Source: CAD feature listing. Evaluate the final solid. Frame: model axes, mm. Face numbers are marked on the shaded views. A direction names the side the tool comes from. Coordinates: 2 decimals unless noted, no trailing zeros. Order: outer loops, then holes, each group sorted by start corner. A loop starts at its lowest first (then second) coordinate and runs counter-clockwise, first axis right, second up. Notation, with made-up numbers: (66, 32.25) -> (77, 32.25) arc R30 ccw to (77, 69.25) -> close; hole circle Ø1 at (26, -12.5). An arc over 180 degrees is marked (long way). Write item = value, one per line. Start each with the question number.
Item 1: Ray query, line 1 along Z through (x, y) = (-9.5, 7.5); line 2 along Y through (x, z) = (13, 20); line 3 along Z through (x, y) = (-51.5, 15.5). Return the intervals inside material, ascending. Write a range as [from, to].
Item 2: Section query C-C (x = 38.5). Output: boundary loops of the cut face in (y, z), then the cut area to 3 significant figures.
Item 3: Contact query for flat-ended pins moving along their axis: pin 1 (2 mm diameter, centred on x = -47.5, z = 14, fed in from -Y); pin 2 (11 mm diameter, centred on y = -25.5, z = 37.5, fed in from -X); pin 3 (7 mm diameter, centred on y = -26, z = 35, fed in from +X); pin 4 (1 mm diameter, centred on x = -15, z = 27, fed in from -Y). Output: stop coordinate, or through.
Item 4: Section query B-B (z = 15). Output: boundary loops of the cut face in (x, y).
Item 5: Section query A-A (y = 15.5). Output: boundary loops of the cut face in (x, z), then the cut area to 3 significant figures.
Item 6: Set-up query: the marked faces 1, 2, 3 and 4. Return all of +Z, -Z, +X, -X, +Y, -Y with unobstructed straight access to the full face (end or side cutting, diameter ignored); none if empty.
Item 7: Section query D-D (y = -4). Output: boundary loops of the cut face in (x, z).
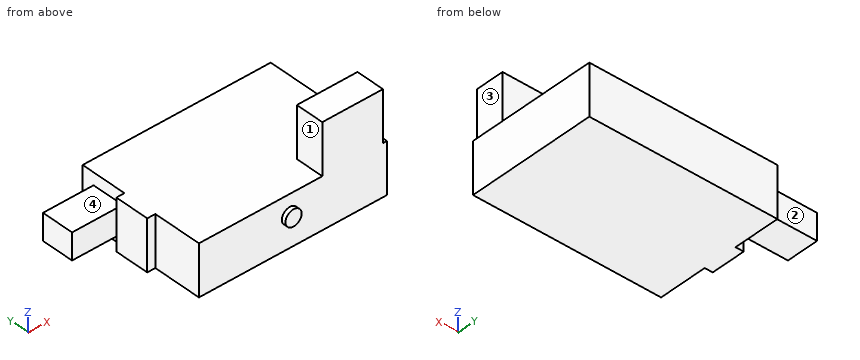
```python
from build123d import *

# Parameters (mm, degrees)
F0_W     = 4
F0_H     = 17
F1_DEPTH = 25
F2_R     = 4
F3_DEPTH = 2
F4_W     = 30
F4_H     = 14
F5_DEPTH = 25
F6_W     = 16
F6_H     = 13
F7_DEPTH = 25


with BuildPart() as f1:
    # F0 (on Top) → F1 (new body)
    with BuildSketch(Plane.XY):
        Polygon((-46.436612, -32), (46.563388, -32), (46.563388, 32), (-46.436612, 32), (-46.436612, 9), (-46.436612, -8), align=None)
        with Locations((-48.436612, 0.5)):
            Rectangle(F0_W, F0_H)
    extrude(amount=F1_DEPTH)

    # F2 (on face) → F3 (join)
    with BuildSketch(Plane.XZ.offset(32)):
        with Locations((-1.436612, 15)):
            Circle(F2_R)
    extrude(amount=F3_DEPTH)

    # F4 (on face) → F5 (join)
    with BuildSketch(Plane.XY.offset(25)):
        with Locations((29.563388, -25)):
            Rectangle(F4_W, F4_H)
    extrude(amount=F5_DEPTH)

    # F6 (on face) → F7 (join)
    with BuildSketch(Plane(origin=(-46.436612, 0, 0), x_dir=(0, -1, 0), z_dir=(-1, 0, 0))):
        with Locations((-18, 12.5)):
            Rectangle(F6_W, F6_H)
    extrude(amount=F7_DEPTH)


solid = f1.part
```
Computed:
q1.line_1 = [0, 25]
q1.line_2 = [-32, 32]
q1.line_3 = [6, 19]
q2.outline = (-32, 0) -> (32, 0) -> (32, 25) -> (-18, 25) -> (-18, 50) -> (-32, 50) -> close
q2.area = 1,950 mm^2
q3.pin_1 = -8
q3.pin_2 = 14.56
q3.pin_3 = 44.56
q3.pin_4 = through
q4.outline = (-71.44, 10) -> (-46.44, 10) -> (-46.44, 9) -> (-50.44, 9) -> (-50.44, -8) -> (-46.44, -8) -> (-46.44, -32) -> (-5.44, -32) -> (-5.44, -34) -> (2.56, -34) -> (2.56, -32) -> (46.56, -32) -> (46.56, 32) -> (-46.44, 32) -> (-46.44, 26) -> (-71.44, 26) -> close
q5.outline = (-71.44, 6) -> (-46.44, 6) -> (-46.44, 0) -> (46.56, 0) -> (46.56, 25) -> (-46.44, 25) -> (-46.44, 19) -> (-71.44, 19) -> close
q5.area = 2,650 mm^2
q6.face_1 = +Z, -X, +Y, -Y
q6.face_2 = +Z, -Z, -X, +Y
q6.face_3 = +Z, +X, +Y, -Y
q6.face_4 = +Z, -X, +Y
q7.outline = (-50.44, 0) -> (46.56, 0) -> (46.56, 25) -> (-50.44, 25) -> close
